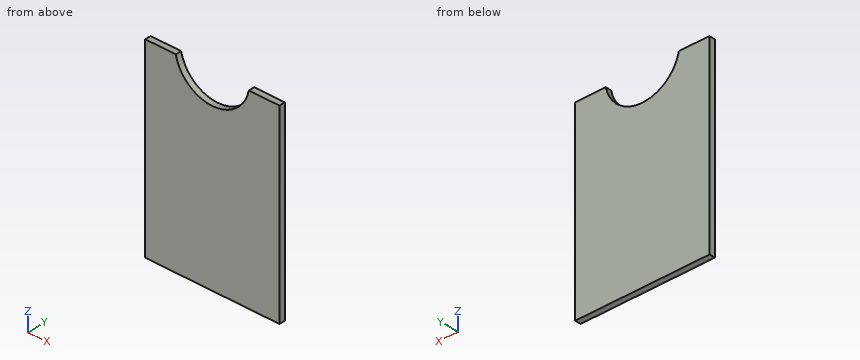
Autodesk Inventor part; units mm, degrees
ref_plane "YZ Plane" through (0, 0, 0) normal (1, 0, 0) x (0, 1, 0)
ref_plane "XZ Plane" through (0, 0, 0) normal (0, 1, 0) x (-1, 0, 0)
ref_plane "XY Plane" through (0, 0, 0) normal (0, 0, 1) x (1, 0, 0)
sketch "Sketch1" plane through (0, 0, 0) normal (0, 1, 0) x (-1, 0, 0)
  line L0 (-45, 65) -> (45, 65)
  line L1 (45, 65) -> (45, -65)
  line L2 (45, -65) -> (-45, -65)
  line L3 (-45, -65) -> (-45, 65)
  line L4 (-45, 65) -> (45, -65) construction
  line L5 (45, 65) -> (-45, -65) construction
  point P0 (0, 0)
  dimension "d1" = 90
  dimension "d2" = 130
extrude "Extrusion1" add sketch "Sketch1" along normal blind 4
sketch "Sketch2" plane through (0, 4, 0) normal (0, 1, 0) x (1, 0, 0)
  line L0 (-45, -65) -> (45, -65)
  arc A0 (24.4949, -65) -> (-24.4949, -65) centre (0, -70) ccw
  line L1 (0, -70) -> (0, 0) construction
  dimension "d5" = 25
  dimension "d6" = 5
extrude "Extrusion2" cut sketch "Sketch2" against normal blind 4
properties part number "Plate 1"
For this review, take the finished solid that the model builds, in its own axes (mm). Coordinates: 2 decimals unless noted, no trailing zeros. Write each loop counter-clockwise with the first axis right and the second up, starting at its lowest first coordinate (ties: lowest second). Pieces come first, ordered by that corner, then holes. Notation, with made-up numbers: (14, -19) - (25, -19) arc R21 cw to (25, -13) - close; hole circle Ø7 at (34, 0). An arc over 180 degrees is marked (long way). Put each result on its own line as item: value.
1. Add section A-A, the plane z = 48. Give the boundary of the cut face in (x, y).
Values found:
outline: (-45, 0) - (-11.87, 0) - (-11.87, 4) - (-45, 4) - close; (11.87, 0) - (45, 0) - (45, 4) - (11.87, 4) - close
2. Add section C-C, the plane x = 17.5. Give the boundary of the cut face in (y, z).
Values found:
outline: (0, -65) - (4, -65) - (4, 52.15) - (0, 52.15) - close
3. Add section B-B, the plane y = 2.7. Give the boundary of the cut face in (x, z), then the cut area to 3 significant figures.
Values found:
outline: (-45, -65) - (45, -65) - (45, 65) - (24.49, 65) arc R25 cw to (-24.49, 65) - (-45, 65) - close
area: 11,000 mm²
4. Add section D-D, the plane x = 2. Give the boundary of the cut face in (y, z).
Values found:
outline: (0, -65) - (4, -65) - (4, 45.08) - (0, 45.08) - close
5. Wall thickness on probe 1 along Z at (x, y) = (6.5, 2.1); probe 2 along Z at (x, y) = (-7, 2.75): over which ranges is each line inside the solid? List them lowest first.
Values found:
probe 1: -65 to 45.86
probe 2: -65 to 46
